Part model, mm, in its own coordinate system. Face numbers are marked on the shaded views. A direction names the side the tool comes from. Coordinates: 2 decimals unless noted, no trailing zeros. Order: outer loops, then holes, each group sorted by start corner. A loop starts at its lowest first (then second) coordinate and runs counter-clockwise, first axis right, second up.
1) Wall check: L1, parallel to Z at x = 22, y = 5; L2, parallel to Y at x = -2, z = 7. Give the ranges that are in metal, low to high.
2) Cut at D-D (x = -11). List the corners of the cut face in (y, z).
3) Cut at C-C (x = 5.5). List the corners of the cut face in (y, z), and give its area (3 significant figures).
4) Cut at B-B (z = 0). List the corners of the cut face in (x, y) (3 decimals).
5) Pin check, flat tips, straight feed: pin 1 Ø16.5 at (x, z) = (-9.5, -8) entering from -Y; pin 2 Ø3.5 at (x, z) = (-22, 24.5) entering from +Y; pin 3 Ø2 at (x, y) = (19, 26.5) entering from -Z. Stop position of each tip, or through.
6) Cut at A-A (y = 51). List the corners of the cut face in (x, z).
7) Tool access for the marked faces 1, 2 and 3: list every direction of +Z, -Z, +X, -X, +Y, -Y with a clear straight run to the whole face (end or side of a thin tool).
```python
from build123d import *

# Parameters (mm, degrees)
F0_R     = 18.75
F1_DEPTH = 1.5
F0_R_2   = 2.5
F2_DEPTH = 7.5
F4_DEPTH = 65
F5_R     = 0.5
F6_R     = 2.875
F7_DEPTH = 20


with BuildPart() as f1:
    # F0 (on Front) → F1 (new body)
    with BuildSketch(Plane.XZ):
        Circle(F0_R)
    extrude(amount=F1_DEPTH)

    # F0 (on Front) → F2 (join)
    with BuildSketch(Plane.XZ):
        with BuildLine():
            Line((25, 27.5), (-25, 27.5))
            ThreePointArc((-25, 27.5), (-26.767766953, 26.767766953), (-27.5, 25))
            Line((-27.5, 25), (-27.5, -25))
            ThreePointArc((-27.5, -25), (-26.767766953, -26.767766953), (-25, -27.5))
            Line((-25, -27.5), (25, -27.5))
            ThreePointArc((25, -27.5), (26.767766953, -26.767766953), (27.5, -25))
            Line((27.5, -25), (27.5, 25))
            ThreePointArc((27.5, 25), (26.767766953, 26.767766953), (25, 27.5))
        make_face()
        with Locations((-22.25, -22.25)):
            Circle(F0_R_2, mode=Mode.SUBTRACT)
        with Locations((22.25, -22.25)):
            Circle(F0_R_2, mode=Mode.SUBTRACT)
        with Locations((-22.25, 22.25)):
            Circle(F0_R_2, mode=Mode.SUBTRACT)
        Circle(F0_R, mode=Mode.SUBTRACT)
        with Locations((22.25, 22.25)):
            Circle(F0_R_2, mode=Mode.SUBTRACT)
        Circle(F0_R)
    extrude(amount=-F2_DEPTH)

    # F3 (on face) → F4 (join)
    with BuildSketch(Plane(origin=(0, 7.5, 0), x_dir=(-1, 0, 0), z_dir=(0, 1, 0))):
        with BuildLine():
            Line((27.5, -17.0038467285), (27.5, 16.874561323))
            Line((27.5, 16.874561323), (22.1223071391, 17.0053998878))
            ThreePointArc((22.1223071391, 17.0053998878), (18.4928159277, 18.5869603521), (17.000002275, 22.253845591))
            Line((17.000002275, 22.253845591), (17.000002275, 27.5))
            Line((17.000002275, 27.5), (-17.000002275, 27.5))
            Line((-17.000002275, 27.5), (-17.000002275, 22.253845591))
            ThreePointArc((-17.000002275, 22.253845591), (-18.5623015375, 18.5132408344), (-22.3232260335, 17.0005115574))
            Line((-22.3232260335, 17.0005115574), (-27.5, 16.874561323))
            Line((-27.5, 16.874561323), (-27.5, -17.0038467285))
            Line((-27.5, -17.0038467285), (-22.4509152226, -17.0038467285))
            ThreePointArc((-22.4509152226, -17.0038467285), (-18.6080321838, -18.4686563976), (-17.000002275, -22.253845591))
            Line((-17.000002275, -22.253845591), (-17.000002275, -27.5))
            Line((-17.000002275, -27.5), (17.000002275, -27.5))
            Line((17.000002275, -27.5), (17.000002275, -22.253845591))
            ThreePointArc((17.000002275, -22.253845591), (18.5376913406, -18.5415357941), (22.2500011375, -17.0038467285))
            Line((22.2500011375, -17.0038467285), (27.5, -17.0038467285))
        make_face()
    extrude(amount=F4_DEPTH)

    # F5
    f5_edges = [f1.edges().sort_by_distance(p)[0] for p in [
        (17.000002, 40, 27.5),
        (-17.000002, 40, 27.5),
        (27.5, 40, -17.003847),
        (27.5, 40, 16.874561),
        (-27.5, 40, 16.874561),
        (-27.5, 40, -17.003847),
        (-17.000002, 40, -27.5),
        (17.000002, 40, -27.5),
    ]]
    fillet(f5_edges, radius=F5_R)

    # F6 (on face) → F7 (join)
    with BuildSketch(Plane.XZ.offset(1.5)):
        Circle(F6_R)
    extrude(amount=F7_DEPTH)


solid = f1.part
```
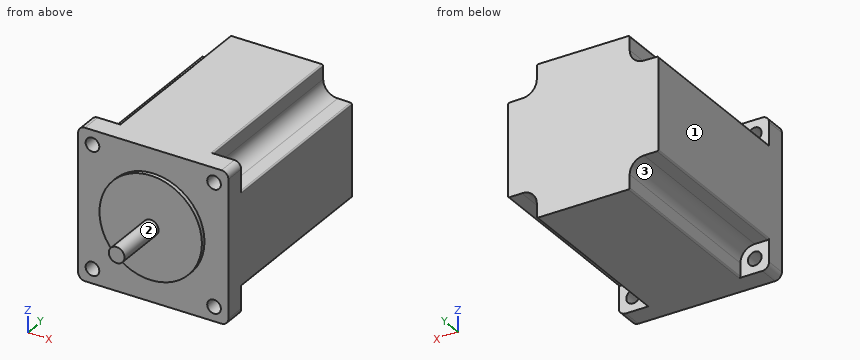
Geometry check:
1. L1: z = -27.5 to -24.74, -19.76 to 19.76, 24.74 to 27.5
1. L2: y = -1.5 to 72.5
2. outline: (-1.5, -15.18) - (0, -15.18) - (0, -27.5) - (72.5, -27.5) - (72.5, 27.5) - (0, 27.5) - (0, 15.18) - (-1.5, 15.18) - close
3. outline: (-1.5, -17.93) - (0, -17.93) - (0, -27.5) - (72.5, -27.5) - (72.5, 27.5) - (0, 27.5) - (0, 17.93) - (-1.5, 17.93) - close
3. area: 4,040 mm2
4. outline: (-27.5, 0) - (-18.75, 0) - (-18.75, -1.5) - (-2.875, -1.5) - (-2.875, -21.5) - (2.875, -21.5) - (2.875, -1.5) - (18.75, -1.5) - (18.75, 0) - (27.5, 0) - (27.5, 72.5) - (-27.5, 72.5) - close
5. pin 1: stops at y = -1.5
5. pin 2: stops at y = 7.5
5. pin 3: stops at z = -19.17
6. outline: (-27.5, -16.5) arc R0.5 ccw to (-27, -17) - (-22.25, -17) arc R5.25 cw to (-17, -22.25) - (-17, -27) arc R0.5 ccw to (-16.5, -27.5) - (16.5, -27.5) arc R0.5 ccw to (17, -27) - (17, -22.25) arc R5.25 cw to (22.45, -17) - (27, -17) arc R0.5 ccw to (27.5, -16.5) - (27.5, 16.39) arc R0.5 ccw to (27.01, 16.89) - (22.32, 17) arc R5.25 cw to (17, 22.25) - (17, 27) arc R0.5 ccw to (16.5, 27.5) - (-16.5, 27.5) arc R0.5 ccw to (-17, 27) - (-17, 22.25) arc R5.25 cw to (-22.12, 17.01) - (-27.01, 16.89) arc R0.5 ccw to (-27.5, 16.39) - close
7. face 1: +Z, -Z, -X, +Y, -Y
7. face 2: -Y
7. face 3: -Z, -X, +Y
